Can you work these out from the model? Positions are in its coordinate system, mm. Face numbers are marked on the shaded views. A direction names the side the tool comes from. Give positions to 0.01 mm unless a question says otherwise; leave off trailing zeros. Loops run counter-clockwise (first coordinate to the right, second up) from the corner with the lowest first, then second, coordinate; pieces in that order, holes last.
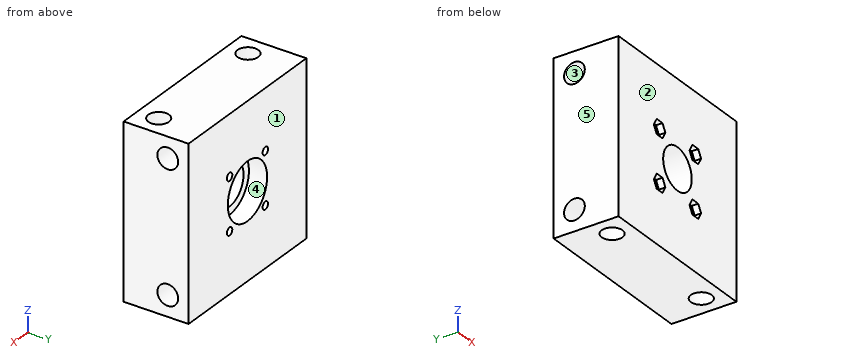
from build123d import *

# Parameters (mm, degrees)
SKETCH1_W           = 66
SKETCH1_H           = 66
SKETCH1_R           = 11
SKETCH1_R_2         = 1.5
BOSS_EXTRUDE1_DEPTH = 25
SKETCH1_4_R         = 11
SKETCH1_4_R_2       = 8
BOSS_EXTRUDE2_DEPTH = 18
SKETCH2_R           = 4
CUT_EXTRUDE1_DEPTH  = 78.910204723
SKETCH3_R           = 4
CUT_EXTRUDE2_DEPTH  = 78.910204723
SKETCH1_5_R         = 1.5
CUT_EXTRUDE3_DEPTH  = 2.5


with BuildPart() as part:
    # Sketch1 → Boss-Extrude1 (new body)
    with BuildSketch(Plane(origin=(0, 0, 0), x_dir=(1, 0, 0), z_dir=(0, 1, 0))):
        Rectangle(SKETCH1_W, SKETCH1_H)
        with Locations(Location((0, 0, 0), (0, 0, 270))):
            Circle(SKETCH1_R, mode=Mode.SUBTRACT)
        with Locations(Location((10, 10, 0), (0, 0, 270))):
            Circle(SKETCH1_R_2, mode=Mode.SUBTRACT)
        with Locations(Location((-10, 10, 0), (0, 0, 270))):
            Circle(SKETCH1_R_2, mode=Mode.SUBTRACT)
        with Locations(Location((10, -10, 0), (0, 0, 270))):
            Circle(SKETCH1_R_2, mode=Mode.SUBTRACT)
        with Locations(Location((-10, -10, 0), (0, 0, 270))):
            Circle(SKETCH1_R_2, mode=Mode.SUBTRACT)
    extrude(amount=BOSS_EXTRUDE1_DEPTH)

    # Sketch1_4 → Boss-Extrude2 (add)
    with BuildSketch(Plane(origin=(0, 0, 0), x_dir=(1, 0, 0), z_dir=(0, 1, 0))):
        with Locations(Location((0, 0, 0), (0, 0, 270))):
            Circle(SKETCH1_4_R)
        with Locations(Location((0, 0, 0), (0, 0, 270))):
            Circle(SKETCH1_4_R_2, mode=Mode.SUBTRACT)
    extrude(amount=BOSS_EXTRUDE2_DEPTH)

    # Sketch2 → Cut-Extrude1 (cut, through all)
    with BuildSketch(Plane.ZY.offset(33)):
        with Locations((-25, 17)):
            Circle(SKETCH2_R)
        with Locations(Location((25, 17, 0), (0, 0, 180))):
            Circle(SKETCH2_R)
    extrude(amount=-CUT_EXTRUDE1_DEPTH, mode=Mode.SUBTRACT)

    # Sketch3 → Cut-Extrude2 (cut, through all)
    with BuildSketch(Plane(origin=(0, 0, -33), x_dir=(-1, 0, 0), z_dir=(0, 0, -1))):
        with Locations((-25, 8)):
            Circle(SKETCH3_R)
        with Locations(Location((25, 8, 0), (0, 0, 180))):
            Circle(SKETCH3_R)
    extrude(amount=-CUT_EXTRUDE2_DEPTH, mode=Mode.SUBTRACT)

    # Sketch1_5 → Cut-Extrude3 (cut)
    # profile 1 of 4: a face of its own
    with BuildSketch(Plane(origin=(0, 0, 0), x_dir=(1, 0, 0), z_dir=(0, 1, 0))):
        Polygon((-11.616580754, -12.8), (-8.383419246, -12.8), (-6.766838493, -10), (-8.383419246, -7.2), (-11.616580754, -7.2), (-13.233161507, -10), align=None)
        with Locations(Location((-10, -10, 0), (0, 0, 270))):
            Circle(SKETCH1_5_R, mode=Mode.SUBTRACT)
    # profile 2 of 4: a face of its own
    with BuildSketch(Plane(origin=(0, 0, 0), x_dir=(1, 0, 0), z_dir=(0, 1, 0))):
        Polygon((-11.616580754, 7.2), (-8.383419246, 7.2), (-6.766838493, 10), (-8.383419246, 12.8), (-11.616580754, 12.8), (-13.233161507, 10), align=None)
        with Locations(Location((-10, 10, 0), (0, 0, 270))):
            Circle(SKETCH1_5_R, mode=Mode.SUBTRACT)
    # profile 3 of 4: a face of its own
    with BuildSketch(Plane(origin=(0, 0, 0), x_dir=(1, 0, 0), z_dir=(0, 1, 0))):
        Polygon((8.383419246, 7.2), (11.616580754, 7.2), (13.233161507, 10), (11.616580754, 12.8), (8.383419246, 12.8), (6.766838493, 10), align=None)
        with Locations(Location((10, 10, 0), (0, 0, 270))):
            Circle(SKETCH1_5_R, mode=Mode.SUBTRACT)
    # profile 4 of 4: a face of its own
    with BuildSketch(Plane(origin=(0, 0, 0), x_dir=(1, 0, 0), z_dir=(0, 1, 0))):
        Polygon((8.383419246, -12.8), (11.616580754, -12.8), (13.233161507, -10), (11.616580754, -7.2), (8.383419246, -7.2), (6.766838493, -10), align=None)
        with Locations(Location((10, -10, 0), (0, 0, 270))):
            Circle(SKETCH1_5_R, mode=Mode.SUBTRACT)
    extrude(amount=CUT_EXTRUDE3_DEPTH, mode=Mode.SUBTRACT)


solid = part.part
(1) Suppose I cut it at B-B on z = -25. List the corners of the cut face in (x, y) for me, plus the area to 3 significant figures.
Returned:
outline: (-33, 0) - (33, 0) - (33, 13) - (-33, 13) - close; (-33, 21) - (33, 21) - (33, 25) - (-33, 25) - close; hole circle Ø8 at (-25, 8); hole circle Ø8 at (25, 8)
area: 1,020 mm2
(2) Thinking about a two-plate mould opening in Y: for the marked faces 1, 2 and 3, which applies, pulls with the +Y half, pulls with the -Y half, needs draft (parallel to the pull), parting line crosses it, or undercut?
Returned:
face 1: pulls with the +Y half
face 2: pulls with the -Y half
face 3: undercut
(3) Suppose I cut it at A-A on x = -25. List the corners of the cut face in (y, z) for me.
Returned:
outline: (0, -33) - (4, -33) - (4, 33) - (0, 33) - close; (12, -33) - (25, -33) - (25, 33) - (12, 33) - close; hole circle Ø8 at (17, -25); hole circle Ø8 at (17, 25)
(4) Which directions (+Z, -Z, +X, -X, +Y, -Y) give clear straight access to the entire face, cutting with the end or side of a thin tool? Please do the marked faces 4 and 5.
Returned:
face 4: +Y
face 5: +Z, -Z, -X, +Y, -Y
(5) Suppose I cut it at C-C on y = 8. List the corners of the cut face in (x, z) for me.
Returned:
outline: (-33, -33) - (-29, -33) - (-29, 33) - (-33, 33) - close; (-21, -33) - (21, -33) - (21, 33) - (-21, 33) - close; (29, -33) - (33, -33) - (33, 33) - (29, 33) - close; hole circle Ø3 at (-10, -10); hole circle Ø3 at (-10, 10); hole circle Ø16 at (0, 0); hole circle Ø3 at (10, -10); hole circle Ø3 at (10, 10)
(6) Suppose I cut it at D-D on x = 10. List the corners of the cut face in (y, z) for me, plus the area to 3 significant figures.
Returned:
outline: (0, -33) - (25, -33) - (25, -11.5) - (2.5, -11.5) - (2.5, -12.8) - (0, -12.8) - close; (0, -7.2) - (2.5, -7.2) - (2.5, -8.5) - (25, -8.5) - (25, -4.58) - (18, -4.58) - (18, 4.58) - (25, 4.58) - (25, 8.5) - (2.5, 8.5) - (2.5, 7.2) - (0, 7.2) - close; (0, 12.8) - (2.5, 12.8) - (2.5, 11.5) - (25, 11.5) - (25, 33) - (0, 33) - close; hole circle Ø8 at (17, -25); hole circle Ø8 at (17, 25)
area: 1,320 mm2
(7) Please list where these lines run through material, in increasing order: probe 1 along X at (y, z) = (15.5, -10); probe 2 along Y at (x, z) = (-25, -13); probe 3 along X at (y, z) = (19.75, 10).
Returned:
probe 1: x = -33 to -11.5, -8.5 to 8.5, 11.5 to 33
probe 2: y = 0 to 4, 12 to 25
probe 3: x = -33 to -11.5, -8.5 to -4.58, 4.58 to 8.5, 11.5 to 33
(8) Will this pin go through, and if not, where does the flat tip stop? P1, Ø4, axis at x = -10, z = 10, coming from the -Y side.
Returned:
P1: stops at y = 2.5
